```python
from build123d import *

# Parameters (mm, degrees)
EXTRUDE_1_DEPTH              = 34
EXTRUDE_START                = 87
SKETCH_4_W                   = 74
SKETCH_4_H                   = 50
EXTRUDE_2_DEPTH              = 5
SKETCH_5_R                   = 25
EXTRUDE_3_DEPTH              = 4
SKETCH_6_R                   = 15.5
EXTRUDE_4_DEPTH              = 3
EXTRUDE_5_DEPTH              = 46
SKETCH_8_W                   = 52
SKETCH_8_H                   = 27
EXTRUDE_6_DEPTH              = 33
EXTRUDE_START_2              = -34
SKETCH_9_R                   = 26
EXTRUDE_7_DEPTH              = 60
CUT_EXTRUDE_1_DEPTH          = 30
SKETCH_11_R                  = 15
CUT_EXTRUDE_2_DEPTH          = 129.611819053
CUT_EXTRUDE_3_REACH          = 148.086
CUT_EXTRUDE_3_END_RADIUS     = 16
SKETCH_12_R                  = 8.5
SKETCH_13_R                  = 13.3
SKETCH_13_R_2                = 9.75
CUT_EXTRUDE_4_DEPTH          = 2.25
HOLE_WIZARD_M6_1_D           = 5
HOLE_WIZARD_M6_1_CSINK_D     = 6.05
HOLE_WIZARD_M6_1_CSINK_ANGLE = 90
HOLE_WIZARD_M6_2_D           = 5
HOLE_WIZARD_M6_2_DEPTH       = 14.497848452
HOLE_WIZARD_M6_2_CSINK_D     = 6.05
HOLE_WIZARD_M6_2_CSINK_ANGLE = 90
HOLE_WIZARD_M6_2_TIP         = 1.502151548
HOLE_WIZARD_M6_3_D           = 5
HOLE_WIZARD_M6_3_DEPTH       = 5
HOLE_WIZARD_M6_3_CSINK_D     = 6.05
HOLE_WIZARD_M6_3_CSINK_ANGLE = 90
HOLE_WIZARD_M10_1_AT_2_COUNT = 2
HOLE_WIZARD_M10_1_AT_2_PITCH = 42


with BuildPart() as part:
    # Sketch 1 → Extrude 1 (new body)
    with BuildSketch(Plane.XY):
        with BuildLine():
            Line((-26, 0), (-26, 60))
            ThreePointArc((-26, 60), (0, 86), (26, 60))
            Line((26, 60), (26, 0))
            ThreePointArc((26, 0), (0, -26), (-26, 0))
        make_face()
    extrude(amount=EXTRUDE_1_DEPTH)

    # Sketch 7 → Extrude 5 (add, symmetric)
    with BuildSketch(Plane(origin=(0, 0, 0), x_dir=(0, 0, -1), z_dir=(1, 0, 0))):
        with BuildLine():
            Line((-27, 60), (-27, 18))
            ThreePointArc((-27, 18), (-17, 8), (-7, 18))
            Line((-7, 18), (-7, 60))
            ThreePointArc((-7, 60), (-17, 70), (-27, 60))
        make_face()
    extrude(amount=EXTRUDE_5_DEPTH, both=True)



with BuildPart() as body_2:
    # Sketch 4 → Extrude 2 (new body)
    with BuildSketch(Plane(origin=(0, 0, 0), x_dir=(1, 0, 0), z_dir=(0, 1, 0)).offset(EXTRUDE_START)):
        with Locations((0, -17)):
            Rectangle(SKETCH_4_W, SKETCH_4_H)
    extrude(amount=EXTRUDE_2_DEPTH)

    # Sketch 5 → Extrude 3 (add)
    with BuildSketch(Plane(origin=(0, 92, 0), x_dir=(1, 0, 0), z_dir=(0, 1, 0))):
        with Locations(Location((0, -17, 0), (0, 0, 270))):
            Circle(SKETCH_5_R)
    extrude(amount=EXTRUDE_3_DEPTH)

    # Sketch 6 → Extrude 4 (add)
    with BuildSketch(Plane(origin=(0, 96, 0), x_dir=(1, 0, 0), z_dir=(0, 1, 0))):
        with Locations(Location((0, -17, 0), (0, 0, 270))):
            Circle(SKETCH_6_R)
    extrude(amount=EXTRUDE_4_DEPTH)


with BuildPart() as part_1:
    add(part.part)

    add(body_2.part)  # Extrude 6 merges body 2
    # Sketch 8 → Extrude 6 (add)
    with BuildSketch(Plane.XY.offset(34)):
        with Locations((0, 73.5)):
            Rectangle(SKETCH_8_W, SKETCH_8_H)
    extrude(amount=-EXTRUDE_6_DEPTH)

    # Sketch 9 → Extrude 7 (add)
    with BuildSketch(Plane.XY.offset(34).offset(EXTRUDE_START_2)):
        Circle(SKETCH_9_R)
    extrude(amount=EXTRUDE_7_DEPTH)

    # Sketch 10 → Cut-Extrude 1 (cut)
    with BuildSketch(Plane(origin=(0, 0, 0), x_dir=(-1, 0, 0), z_dir=(0, 0, -1))):
        with BuildLine():
            Line((-16, 0), (-16, 60))
            ThreePointArc((-16, 60), (0, 76), (16, 60))
            Line((16, 60), (16, 0))
            ThreePointArc((16, 0), (0, -16), (-16, 0))
        make_face()
    extrude(amount=-CUT_EXTRUDE_1_DEPTH, mode=Mode.SUBTRACT)

    # Sketch 11 → Cut-Extrude 2 (cut, through all)
    with BuildSketch(Plane.XY.offset(60)):
        Circle(SKETCH_11_R)
    extrude(amount=-CUT_EXTRUDE_2_DEPTH, mode=Mode.SUBTRACT)

    # Cut-Extrude 3: up to this cylinder (the profile starts outside it)
    cut_extrude_3_end = Plane(origin=(0, 60, 17), z_dir=(0, 0, -1)) * Cylinder(CUT_EXTRUDE_3_END_RADIUS, 329.172, mode=Mode.PRIVATE)
    # Sketch 12 → Cut-Extrude 3 (cut, up to the surface)
    with BuildSketch(Plane(origin=(0, 99, 0), x_dir=(1, 0, 0), z_dir=(0, 1, 0)), mode=Mode.PRIVATE) as cut_extrude_3_sk1:
        with Locations(Location((0, -17, 0), (0, 0, 270))):
            Circle(SKETCH_12_R)
    cut_extrude_3_tool1 = extrude(cut_extrude_3_sk1.sketch, amount=-CUT_EXTRUDE_3_REACH, mode=Mode.PRIVATE) - cut_extrude_3_end
    add(cut_extrude_3_tool1.solids().sort_by_distance((0, 99, 17))[0], mode=Mode.SUBTRACT)

    # Sketch 13 → Cut-Extrude 4 (cut)
    with BuildSketch(Plane(origin=(0, 99, 0), x_dir=(1, 0, 0), z_dir=(0, 1, 0))):
        with Locations(Location((0, -17, 0), (0, 0, 270))):
            Circle(SKETCH_13_R)
        with Locations(Location((0, -17, 0), (0, 0, 270))):
            Circle(SKETCH_13_R_2, mode=Mode.SUBTRACT)
    extrude(amount=-CUT_EXTRUDE_4_DEPTH, mode=Mode.SUBTRACT)

    # Hole Wizard M6 _1 (through all)
    with Locations(Plane(origin=(0, 96, 0), x_dir=(1, 0, 0), z_dir=(0, 1, 0))):
        with Locations((0, 3)):
            CounterSinkHole(HOLE_WIZARD_M6_1_D / 2, HOLE_WIZARD_M6_1_CSINK_D / 2, counter_sink_angle=HOLE_WIZARD_M6_1_CSINK_ANGLE)

    # Hole Wizard M6 _2
    with Locations(Plane(origin=(0, 96, 0), x_dir=(1, 0, 0), z_dir=(0, 1, 0))):
        with Locations((17.320508076, -27), (-17.320508076, -27)):
            CounterSinkHole(HOLE_WIZARD_M6_2_D / 2, HOLE_WIZARD_M6_2_CSINK_D / 2, depth=HOLE_WIZARD_M6_2_DEPTH, counter_sink_angle=HOLE_WIZARD_M6_2_CSINK_ANGLE)
            with Locations((0, 0, -(HOLE_WIZARD_M6_2_DEPTH + HOLE_WIZARD_M6_2_TIP / 2))):  # 118° drill point
                Cone(0, HOLE_WIZARD_M6_2_D / 2, HOLE_WIZARD_M6_2_TIP, mode=Mode.SUBTRACT)

    # Hole Wizard M6 _3
    with Locations(Plane(origin=(0, 92, 0), x_dir=(1, 0, 0), z_dir=(0, 1, 0))):
        with Locations((30, -1), (0, -17), (-30, -1), (-30, -33), (30, -33)):
            CounterSinkHole(HOLE_WIZARD_M6_3_D / 2, HOLE_WIZARD_M6_3_CSINK_D / 2, depth=HOLE_WIZARD_M6_3_DEPTH, counter_sink_angle=HOLE_WIZARD_M6_3_CSINK_ANGLE)

    # Sketch 21 → Hole Wizard M10 _1 (revolve, cut)
    with BuildSketch(Plane(origin=(46, 60, 17), x_dir=(0, 0, -1), z_dir=(0, 1, 0))):
        Polygon((0, 0), (0, 22), (4.25, 19.446342369), (4.25, 0.775), (5.025, 0), align=None)
    hole_wizard_m10_1 = revolve(axis=Axis((52.35, 60, 17), (-1, 0, 0)), mode=Mode.SUBTRACT)

    # Hole Wizard M10 _1 at 2: Hole Wizard M10 _1 ×2
    with Locations(*[(0, -i * HOLE_WIZARD_M10_1_AT_2_PITCH, 0) for i in range(1, HOLE_WIZARD_M10_1_AT_2_COUNT)]):
        add(hole_wizard_m10_1, mode=Mode.SUBTRACT)

    # Mirror 1: Hole Wizard M10 _1 across plane
    add(hole_wizard_m10_1.mirror(Plane(origin=(0, 0, 0), x_dir=(0, 0, 1), z_dir=(1, 0, 0))), mode=Mode.SUBTRACT)

    # Mirror 1 copy 1 sketch → Mirror 1 copy 1 (revolve, cut)
    with BuildSketch(Plane(origin=(-46, 18, 17), x_dir=(0, 0, -1), z_dir=(0, 1, 0))):
        Polygon((0, 0), (0, -22), (4.25, -19.446342369), (4.25, -0.775), (5.025, 0), align=None)
    revolve(axis=Axis((-52.35, 18, 17), (-1, 0, 0)), mode=Mode.SUBTRACT)


solid = part_1.part
```
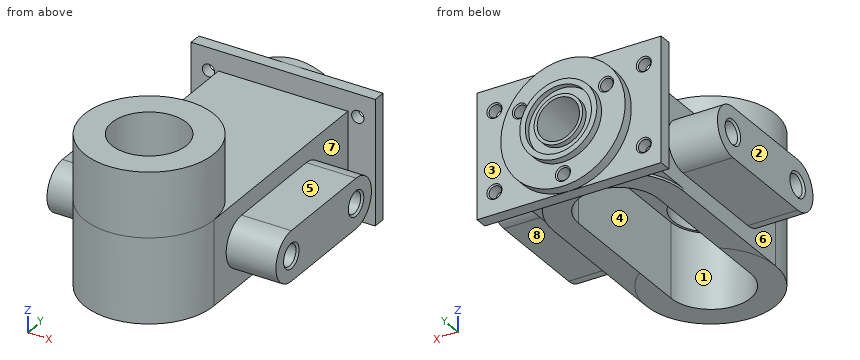
Can you work these out from the model? Positions are in its coordinate system, mm. Face numbers are marked on the shaded views. A direction names the side the tool comes from. Round coordinates to 2 decimals unless told otherwise and drop trailing zeros. Loops run counter-clockwise (first coordinate to the right, second up) from the corner with the lowest first, then second, coordinate; pieces in that order, holes last. Notation, with made-up numbers: M 14.25,18.5 L 36.25,18.5 A10 cw 36.25,27.5 Z; hole C -31.75,36.25 d5. An arc over 180 degrees is marked long. Answer in a Markdown table with one row per item.
1. I'm going to push flat-ended pins straight in: pin 1 Ø3 at (x, z) = (36.5, -0.5) entering from +Y; pin 2 Ø1 at (x, y) = (19, 86) entering from -Z; pin 3 Ø11 at (x, z) = (-21.5, 7.5) entering from +Y. Where does each tip first touch, or does it pass through?
Established:
| item | result |
|---|---|
| pin 1 | y = 92 |
| pin 2 | z = 1 |
| pin 3 | y = 96 |
2. If we section it at A-A, the plane x = -30: Please give me the cut outline in (y, z) (3 decimals), plus the area to 3 significant figures.
Established:
| item | result |
|---|---|
| outline | M 18,7 L 60,7 A10 ccw 60,27 L 18,27 A10 ccw Z; M 87,-8 L 92,-8 L 92,-2.025 L 91.475,-1.5 L 87,-1.5 Z; M 87,3.5 L 91.475,3.5 L 92,4.025 L 92,29.975 L 91.475,30.5 L 87,30.5 Z; M 87,35.5 L 91.475,35.5 L 92,36.025 L 92,42 L 87,42 Z; hole C 18,17 d8.5; hole C 60,17 d8.5 |
| area | 1,240 mm² |
3. If we section it at B-B, the plane y = -2: Please give me the cut outline in (x, z).
Established:
| item | result |
|---|---|
| outline | M -25.92,0 L -15.87,0 L -15.87,30 L -14.87,30 L -14.87,60 L -25.92,60 Z; M 14.87,30 L 15.87,30 L 15.87,0 L 25.92,0 L 25.92,60 L 14.87,60 Z |
4. On a 3-axis mill with a long thin cutter (end or side, diameter ignored), from which of +Z, -Z, +X, -X, +Y, -Y can I reach the whole of each face in a straight line? I mean the marked faces 4, 5, 6, 7 and 8. Say none if no direction works.
Established:
| item | result |
|---|---|
| face 4 | -Z |
| face 5 | +Z, +X, -Y |
| face 6 | -X |
| face 7 | +X |
| face 8 | -Z, +X, -Y |
5. Please list where these lines run through material, in increasing order: line 1 (X direction, y = 88.7, z = 33); line 2 (X direction, y = 88, z = 27); line 3 (Z direction, x = -30, y = 90.35). Write a range as from..to.
Established:
| item | result |
|---|---|
| line 1 | -37..-32.5, -27.5..27.5, 32.5..37 |
| line 2 | -37..-19.82, -14.82..14.82, 19.82..37 |
| line 3 | -8..-1.5, 3.5..30.5, 35.5..42 |
6. If we section it at C-C, the plane y = 49.5: Please give me the cut outline in (x, z), plus the area to 3 significant figures.
Established:
| item | result |
|---|---|
| outline | M -46,7 L -26,7 L -26,0 L -16,0 L -16,30 L 16,30 L 16,0 L 26,0 L 26,7 L 46,7 L 46,27 L 26,27 L 26,34 L -26,34 L -26,27 L -46,27 Z |
| area | 1,610 mm² |
7. If we section it at D-D, the plane z = 46: Please give me the cut outline in (x, y), plus the area to 3 significant figures.
Established:
| item | result |
|---|---|
| outline | C 0,0 d52; hole C 0,0 d30 |
| area | 1,420 mm² |
8. Thinking about a two-plate mould opening in Y: for the marked faces 1, 2 and 3, which applies, pulls with the +Y half, pulls with the -Y half, needs draft (parallel to the pull), parting line crosses it, or undercut?
Established:
| item | result |
|---|---|
| face 1 | undercut |
| face 2 | needs draft |
| face 3 | pulls with the +Y half |
